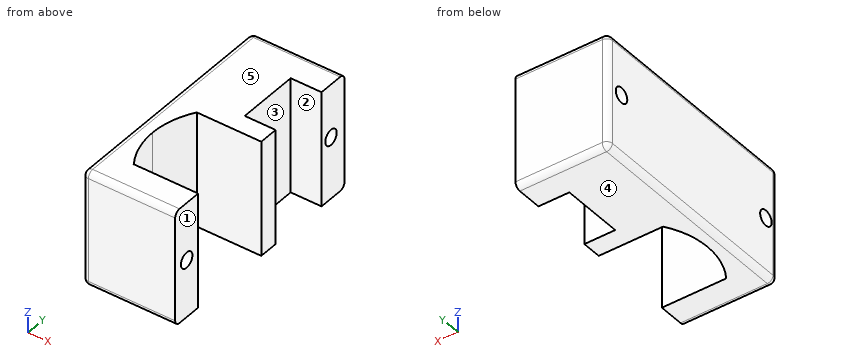
Autodesk Fusion 360 part; units mm, degrees
sketch "Esboço1" plane through (0, 0, 0) normal (0, 0, 1) x (1, 0, 0)
  line L0 (-3.0001, 62) -> (21, 62)
  line L1 (21, 62) -> (21, 54)
  line L2 (21, 54) -> (13, 54)
  line L3 (13, 54) -> (13, 38)
  line L4 (13, 38) -> (21, 38)
  line L5 (21, 11) -> (21, 3)
  line L6 (-3, 3) -> (-3, 62)
  line L7 (-3, 3) -> (21, 3)
  line L8 (21, 33) -> (21, 38)
  line L9 (-3.0001, 62) -> (-3, 62)
  line L10 (21, 33) -> (1, 33)
  line L11 (1, 11) -> (21, 11)
  arc A0 (1, 22) -> (4.2967, 11) centre (21, 22) ccw
  arc A1 (4.2967, 33) -> (1, 22) centre (21, 22) ccw
  dimension "d2" = 16
  dimension "d3" = 8
  dimension "d5" = 8
  dimension "d8" = 8
  dimension "d10" = 8
  dimension "d35" = 5
  dimension "d36" = 24
extrude "Extrusão1" add sketch "Esboço1" along normal blind 30
hole "Furo2" at (-3, 7, 15) direction (1, 0, 0) diameter 4 depth 25 tip angle 180
hole "Furo3" at (-3, 57.307, 16.094) direction (1, 0, 0) diameter 4 depth 25 tip angle 180
fillet "Arredondamento4" radius 1.5 8 edges at (9, 62, 30) (-3, 62, 15) (-3, 32.5, 30) (-3, 32.5, 0) (-3, 3, 15) (9, 3, 0) (9, 3, 30) (9, 62, 0)
Geometry: final body of the model. Coordinates: model frame, mm. Face numbers are marked on the shaded views. A direction names the side the tool comes from. Coordinates: 2 decimals unless noted, no trailing zeros. Order: outer loops, then holes, each group sorted by start corner. A loop starts at its lowest first (then second) coordinate and runs counter-clockwise, first axis right, second up. Notation, with made-up numbers: (50.25, -16) -> (79.25, -16) arc R33 ccw to (79.25, 20) -> close; hole circle Ø8 at (85, 86). An arc over 180 degrees is marked (long way). Write item = value, one per line.
(1) Line query: line 1 (Y direction, x = 14.5, z = 18.5); line 2 (Y direction, x = 11.75, z = 11); line 3 (Z direction, x = 15.25, y = 7). Output: solid intervals per line, ascending.
Solved:
line_1 = 3 to 11, 33 to 38, 54 to 62
line_2 = 3 to 11, 33 to 62
line_3 = 0 to 13, 17 to 30
(2) Cut plane A-A on x = 16. Return loops of the section in (y, z), plus the area to 3 significant figures.
Solved:
outline = (3, 1.5) arc R1.5 ccw to (4.5, 0) -> (11, 0) -> (11, 30) -> (4.5, 30) arc R1.5 ccw to (3, 28.5) -> close; (33, 0) -> (38, 0) -> (38, 30) -> (33, 30) -> close; (54, 0) -> (60.5, 0) arc R1.5 ccw to (62, 1.5) -> (62, 28.5) arc R1.5 ccw to (60.5, 30) -> (54, 30) -> close; hole circle Ø4 at (7, 15); hole circle Ø4 at (57.31, 16.09)
area = 603 mm²
(3) Pull-direction query (Z, two-part tool) for the marked faces 3, 4 and 5; classes: pulls with the +Z half, pulls with the -Z half, needs draft (parallel to the pull), parting line crosses it, or undercut.
Solved:
face_3 = needs draft
face_4 = pulls with the -Z half
face_5 = pulls with the +Z half
(4) Cut plane B-B on z = 15. Return loops of the section in (x, y).
Solved:
outline = (-3, 4.5) arc R1.5 ccw to (-1.5, 3) -> (21, 3) -> (21, 5) -> (-3, 5) -> close; (-3, 9) -> (21, 9) -> (21, 11) -> (4.3, 11) arc R20 cw to (1, 22) arc R20 cw to (4.3, 33) -> (21, 33) -> (21, 38) -> (13, 38) -> (13, 54) -> (21, 54) -> (21, 55.63) -> (-3, 55.63) -> close; (-3, 58.98) -> (21, 58.98) -> (21, 62) -> (-1.5, 62) arc R1.5 ccw to (-3, 60.5) -> close
(5) Access query for the marked faces 1 and 2. Directions: +Z, -Z, +X, -X, +Y, -Y. A direction counts if a zero-diameter tool reaches every point of the face in a straight line with its end or side. Return the directions, or none.
Solved:
face_1 = +Z, -Z, +X, +Y, -Y
face_2 = +Z, -Z, +X
(6) Cut plane C-C on z = 25.25. Return loops of the section in (x, y), plus the area to 3 significant figures.
Solved:
outline = (-3, 4.5) arc R1.5 ccw to (-1.5, 3) -> (21, 3) -> (21, 11) -> (4.3, 11) arc R20 cw to (1, 22) arc R20 cw to (4.3, 33) -> (21, 33) -> (21, 38) -> (13, 38) -> (13, 54) -> (21, 54) -> (21, 62) -> (-1.5, 62) arc R1.5 ccw to (-3, 60.5) -> close
area = 870 mm²
